For this review, take the finished solid that the model builds, in its own axes (mm). A direction names the side the tool comes from. Coordinates: 2 decimals unless noted, no trailing zeros. Loops run counter-clockwise (first coordinate to the right, second up) from the corner with the lowest first, then second, coordinate; pieces in that order, holes last. Notation, with made-up numbers: (22, 40.5) - (80, 40.5) arc R16 ccw to (80, 67.5) - close; hole circle Ø4 at (18, 33). An arc over 180 degrees is marked (long way). Answer as a JSON object with one key per item and string values. Group by question number.
Item 1: Clearance check with flat-ended pins moving along their axes: pin 1 (4 mm diameter, centred on x = 11, y = 6, fed in from +Z); pin 2 (18.5 mm diameter, centred on x = 16.44, z = -21.09, fed in from +Y); pin 3 (1 mm diameter, centred on x = 21, z = -8.5, fed in from +Y). State where each tip first meets the part, or that it passes through.
Item 2: Tool access review of faces 4 (the flat face through (0, 1, -18)), 5 (the flat face through (17, 4, -21)): name each direction out of +Z, -Z, +X, -X, +Y, -Y from which nothing blocks a thin tool from reaching the whole face with its end or side.
Item 3: We need section B-B (z = -7). Give the boundary of the cut face in (x, y), then the cut area to 3 significant figures.
Item 4: Mouldability with a two-part tool opening along X and no side actions: class faces 1 (the cylindrical face through (26.139, 6.535, -14.912)), 2 (the cylindrical face through (15.95, 5.45, -8.68)), 3 (the flat face through (16, 1, 0)) as released by +X, released by -X, zero draft, split by the parting line, or undercut.
Item 5: We need section A-A (x = 13.5). Give the boundary of the cut face in (y, z), then the cut area to 3 significant figures.
Item 6: We need section D-D (y = 6). Give the boundary of the cut face in (x, z).
Item 7: We need section C-C (y = 2.75). Give the boundary of the cut face in (x, z).
Item 8: To check wall thickness, follow line 1 (X direction, y = 8, z = -21.5); line 2 (X direction, y = 4.25, z = -21); line 3 (Y direction, x = 25, z = -25). State the ranges of each line that lie inside material, in increasing order.
from build123d import *

# Parameters (mm, degrees)
SKETCH_1_W          = 32
SKETCH_1_H          = 36
EXTRUDE_1_DEPTH     = 2
FILLET_3_R          = 0.5
SKETCH_2_R          = 12.5
EXTRUDE_2_DEPTH     = 7
SKETCH_3_R          = 11.5
SKETCH_3_R_2        = 0.070206985
CUT_EXTRUDE_1_DEPTH = 5


with BuildPart() as part:
    # 草图1 → 凸台-拉伸1 (new body)
    with BuildSketch(Plane(origin=(0, 0, 0), x_dir=(1, 0, 0), z_dir=(0, 1, 0))):
        with Locations((16, 18)):
            Rectangle(SKETCH_1_W, SKETCH_1_H)
    extrude(amount=EXTRUDE_1_DEPTH)

    # 圆角3
    fillet_3_edges = [part.edges().sort_by_distance(p)[0] for p in [
        (32, 2, -18),
        (16, 2, -36),
        (0, 2, -18),
        (16, 2, 0),
    ]]
    fillet(fillet_3_edges, radius=FILLET_3_R)

    # 草图2 → 凸台-拉伸2 (add)
    with BuildSketch(Plane(origin=(0, 2, 0), x_dir=(1, 0, 0), z_dir=(0, 1, 0))):
        with Locations(Location((16.5, 21.167902567, 0), (0, 0, 90))):
            Circle(SKETCH_2_R)
    extrude(amount=EXTRUDE_2_DEPTH)

    # 草图3 → 切除-拉伸1 (cut)
    with BuildSketch(Plane(origin=(0, 9, 0), x_dir=(1, 0, 0), z_dir=(0, 1, 0))):
        with Locations(Location((16.442109052, 21.094763366, 0), (0, 0, 270))):
            Circle(SKETCH_3_R)
        with Locations((0, 24.191575331)):
            Circle(SKETCH_3_R_2)
    extrude(amount=-CUT_EXTRUDE_1_DEPTH, mode=Mode.SUBTRACT)


solid = part.part
Check sheet entries:
{
 "1": {"pin 1": "stops at z = -9.17", "pin 2": "stops at y = 4", "pin 3": "stops at y = 2"},
 "2": {"face 4": "+Z, -Z, -X, +Y, -Y", "face 5": "+Y"},
 "3": {"outline": "(0, 0) - (32, 0) - (32, 1.5) arc R0.5 ccw to (31.5, 2) - (0.5, 2) arc R0.5 ccw to (0, 1.5) - close", "area": "63.9 mm2"},
 "4": {"face 1": "undercut", "face 2": "split by the parting line", "face 3": "zero draft"},
 "5": {"outline": "(0, -36) - (1.5, -36) arc R0.5 ccw to (2, -35.5) - (2, -33.3) - (9, -33.3) - (9, -32.21) - (4, -32.21) - (4, -9.98) - (9, -9.98) - (9, -9.03) - (2, -9.03) - (2, -0.5) arc R0.5 ccw to (1.5, 0) - (0, 0) - close", "area": "131 mm2"},
 "6": {"outline": "circle Ø25 at (16.5, -21.17); hole circle Ø23 at (16.44, -21.09)"},
 "7": {"outline": "circle Ø25 at (16.5, -21.17)"},
 "8": {"line 1": "x = 4 to 4.95, 27.93 to 29", "line 2": "x = 4 to 4.94, 27.94 to 29", "line 3": "y = 0 to 4"}
}
